from build123d import *

# Parameters (mm, degrees)
SKETCH1_W           = 12.7
SKETCH1_H           = 271.365530146
BOSS_EXTRUDE1_DEPTH = 248.25
SKETCH2_W           = 172.05
SKETCH2_H           = 118.965530146
CUT_EXTRUDE1_DEPTH  = 13.7
FILLET1_R           = 50.8
HOLE1_D             = 3.175
HOLE1_DEPTH         = 31.75
HOLE1_CSINK_D       = 10.16
HOLE1_CSINK_ANGLE   = 82
HOLE1_TIP           = 0.953866233
HOLE2_D             = 3.175
HOLE2_DEPTH         = 31.75
HOLE2_CSINK_D       = 10.16
HOLE2_CSINK_ANGLE   = 82
HOLE2_TIP           = 0.953866233
HOLE3_D             = 3.175
HOLE3_DEPTH         = 31.75
HOLE3_CSINK_D       = 10.16
HOLE3_CSINK_ANGLE   = 82
HOLE3_TIP           = 0.953866233


with BuildPart() as part:
    # Sketch1 → Boss-Extrude1 (new body)
    with BuildSketch(Plane.XY):
        with Locations((-228.402967181, -52.841023691)):
            Rectangle(SKETCH1_W, SKETCH1_H)
    extrude(amount=BOSS_EXTRUDE1_DEPTH)

    # Sketch2 → Cut-Extrude1 (cut, through all)
    with BuildSketch(Plane.ZY.offset(234.752967181)):
        with Locations((124.125, -52.841023691)):
            Rectangle(SKETCH2_W, SKETCH2_H)
    extrude(amount=-CUT_EXTRUDE1_DEPTH, mode=Mode.SUBTRACT)

    # Fillet1
    fillet1_edges = [part.edges().sort_by_distance(p)[0] for p in [
        (-228.402967181, 6.641741382, 210.15),
        (-228.402967181, -112.323788764, 210.15),
        (-228.402967181, -112.323788764, 38.1),
        (-228.402967181, 6.641741382, 38.1),
    ]]
    fillet(fillet1_edges, radius=FILLET1_R)

    # Hole1
    with Locations(Plane(origin=(181.039434513, -52.974999997, -12.7), x_dir=(0, -1, 0), z_dir=(0, 0, -1))):
        with Locations((129.198788767, 384.042401694), (-129.466741379, 384.042401694), (-129.466741379, 304.786761906), (-110.416741379, 409.442401694), (-0.133976306, 409.442401694), (110.148788767, 409.442401694), (129.198788767, 304.786761906)):
            CounterSinkHole(HOLE1_D / 2, HOLE1_CSINK_D / 2, depth=HOLE1_DEPTH, counter_sink_angle=HOLE1_CSINK_ANGLE)
            with Locations((0, 0, -(HOLE1_DEPTH + HOLE1_TIP / 2))):  # 118° drill point
                Cone(0, HOLE1_D / 2, HOLE1_TIP, mode=Mode.SUBTRACT)

    # Hole2
    with Locations(Plane(origin=(-234.752967181, -52.974999997, -1090.512770337), x_dir=(0, -1, 0), z_dir=(-1, 0, 0))):
        with Locations((-129.466741379, 1300.662770337), (-129.466741379, 1128.612770337), (129.198788767, 1128.612770337), (129.198788767, 1300.662770337)):
            CounterSinkHole(HOLE2_D / 2, HOLE2_CSINK_D / 2, depth=HOLE2_DEPTH, counter_sink_angle=HOLE2_CSINK_ANGLE)
            with Locations((0, 0, -(HOLE2_DEPTH + HOLE2_TIP / 2))):  # 118° drill point
                Cone(0, HOLE2_D / 2, HOLE2_TIP, mode=Mode.SUBTRACT)

    # Hole3
    with Locations(Plane(origin=(-222.052967181, -52.974999997, -1090.512770337), x_dir=(0, 1, 0), z_dir=(1, 0, 0))):
        with Locations((-100.332047386, 1313.362770337), (100.599999997, 1313.362770337), (100.599999997, 1115.912770337), (100.599999997, 1214.637770337), (-100.332047386, 1214.637770337), (-100.332047386, 1115.912770337)):
            CounterSinkHole(HOLE3_D / 2, HOLE3_CSINK_D / 2, depth=HOLE3_DEPTH, counter_sink_angle=HOLE3_CSINK_ANGLE)
            with Locations((0, 0, -(HOLE3_DEPTH + HOLE3_TIP / 2))):  # 118° drill point
                Cone(0, HOLE3_D / 2, HOLE3_TIP, mode=Mode.SUBTRACT)


solid = part.part
Part model, mm, in its own coordinate system. A direction names the side the tool comes from. Give positions to 0.01 mm unless a question says otherwise; leave off trailing zeros. Order: outer loops, then holes, each group sorted by start corner. A loop starts at its lowest first (then second) coordinate and runs counter-clockwise, first axis right, second up. Notation, with made-up numbers: (29.25, -21) - (44.25, -21) arc R22 cw to (44.25, -3) - close; hole circle Ø6 at (31.5, 73). An arc over 180 degrees is marked (long way). One line per question, with ' | ' between items.
1. Drop flat-ended pins along their axis: P1, Ø4, axis at y = 76.49, z = 38.1, coming from the +X side; P2, Ø4, axis at y = -182.17, z = 38.1, coming from the -X side; P3, Ø4, axis at y = -153.31, z = 25.4, coming from the +X side; P4, Ø2.5, axis at y = 47.625, z = 25.4, coming from the -X side. Give the stop position or say it passes through.
Filled in:
P1: x = -222.05 | P2: x = -231.21 | P3: x = -225.59 | P4: through
2. Band-saw the part on A-A on z = 101. List the corners of the cut face in (x, y).
Filled in:
outline: (-234.75, -188.52) - (-222.05, -188.52) - (-222.05, -112.32) - (-234.75, -112.32) - close; (-234.75, 6.64) - (-222.05, 6.64) - (-222.05, 82.84) - (-234.75, 82.84) - close
3. Pull direction Z, two halves, no side cores. Call faces 1 (the face through (-230.93, 78.168, 38.628)), 2 (the face through (-228, -51, 248.25)), 3 (the face through (-228, 82.842, 122)): +Z half, -Z half, draft (parallel to the pull), parting line (faces both ways), or undercut.
Filled in:
face 1: undercut | face 2: +Z half | face 3: draft
4. Band-saw the part on B-B on y = -15.5. List the corners of the cut face in (x, z), then the cut area to 3 significant figures.
Filled in:
outline: (-234.75, 0) - (-222.05, 0) - (-222.05, 46.96) - (-234.75, 46.96) - close; (-234.75, 201.29) - (-222.05, 201.29) - (-222.05, 248.25) - (-234.75, 248.25) - close | area: 1,190 mm²
5. Which spindle directions (+Z, -Z, +X, -X, +Y, -Y) get a long thin tool onto all of the face, cutting with end or side? Do faces 4 (the face through (-222.053, -115, 122)), 5 (the face through (-228, -112.324, 124)). Say none if no direction does.
Filled in:
face 4: +Z, -Z, +X, +Y, -Y | face 5: +X, -X
6. Drill centre lines: probe 1 along Y at (x, z) = (-224, 106.5); probe 2 along Y at (x, z) = (-231.5, 221.5); probe 3 along Z at (x, y) = (-222.75, -56). Where is each one in solid material? Low to high.
Filled in:
probe 1: -188.52 to -112.32, 6.64 to 82.84 | probe 2: -188.52 to -154.14, -152.47 to 46.79, 48.46 to 82.84 | probe 3: 0 to 38.1, 210.15 to 248.25
